Read the model definition and answer for the solid it produces. Units are mm, in the model's axes. A direction names the side the tool comes from. Round coordinates to 2 decimals unless told otherwise and drop trailing zeros. Write each loop counter-clockwise with the first axis right and the second up, starting at its lowest first coordinate (ties: lowest second). Pieces come first, ordered by that corner, then holes. Notation, with made-up numbers: (42, 56.25) - (101, 56.25) arc R21 ccw to (101, 72.25) - close; hole circle Ø6 at (-33.75, -0.75). An arc over 180 degrees is marked (long way). Use one line per item in the form item = value. Start each with the question number.
1) Consider line 1 along X through (y, z) = (44.5, -8.5); line 2 along Y through (x, z) = (41, 7.25); line 3 along X through (y, z) = (43, 2.5). Determine where each line is inside the solid, lowest interval first. Write a range as from..to.
2) For faces 5 (the face through (8, 11, -4)), 6 (the face through (20, 57, 7)), 7 (the face through (32, 11, -4)), 8 (the face through (30, 6, 4)), 9 (the face through (28.11, 47.03, -1.64)), determine the directions among +Z, -Z, +X, -X, +Y, -Y from which every point of the face is accessible in a straight line to the end or side of a thin tool.
3) The part is cut by section A-A, the plane z = 8.25. Give the vertices of the cut face in (x, y).
4) Each of these flat-tipped pins is pushed along its axis until it touches: pin 1 (10 mm diameter, centred on y = 27, z = -4.5, fed in from +X); pin 2 (12 mm diameter, centred on x = 39, y = 54, fed in from -Z); pin 3 (17.5 mm diameter, centred on x = 23.5, y = 32, fed in from +Z). Where does it stop, or does it pass through?
5) For a pull along Y with two mould halves and no side action, classify faces 1 (the face through (30.78, 35.27, -8.04)), 2 (the face through (19.9, 0, 7.2)), 3 (the face through (20, 60, 8)), 4 (the face through (20, 3, 7)) as released by +Y, released by -Y, zero draft, split by the parting line, or undercut.
6) The part is cut by section B-B, the plane x = -5. Count the separate pieces of the cut face and the enclosed holes in it, plus the area to 3 significant figures.
7) The part is cut by section C-C, the plane z = -6.5. Give the vertices of the cut face in (x, y).
from build123d import *

# Parameters (mm, degrees)
CYLINDER002003_R     = 2
CYLINDER002003_DEPTH = 30
CYLINDER002004_R     = 3
CYLINDER002004_DEPTH = 11
CYLINDER_W           = 10
CYLINDER_H           = 31
CYLINDER_ANGLE       = 180
CYLINDER_ROLL_ANGLE  = -90
CYLINDER002006_R     = 10
CYLINDER002006_DEPTH = 6
SPHERE001_ROLL_ANGLE = 1
BOX008_W             = 20
BOX008_H             = 31
BOX008_DEPTH         = 6
CYLINDER006_R        = 2
CYLINDER006_DEPTH    = 10
CYLINDER008_R        = 2
CYLINDER008_DEPTH    = 10
CYLINDER007_R        = 2
CYLINDER007_DEPTH    = 10
CYLINDER005_R        = 2
CYLINDER005_DEPTH    = 10
CYLINDER001_R        = 12
CYLINDER001_DEPTH    = 12
BOX003_W             = 24
BOX003_H             = 30
BOX003_DEPTH         = 18
BOX_W                = 60
BOX_H                = 60
BOX_DEPTH            = 3
CYLINDER002002_R     = 5
CYLINDER002002_DEPTH = 15


with BuildPart() as obj1:
    # Cylinder002003 → Cylinder002003 (new body)
    with BuildSketch(Plane(origin=(26.5, 44.5, -13), x_dir=(1, 0, 0), z_dir=(0, 0, 1))):
        Circle(CYLINDER002003_R)
    extrude(amount=CYLINDER002003_DEPTH)


with BuildPart() as schnittkegel:
    # Cone003 → Cone003 (revolve)
    with BuildSketch(Plane(origin=(20, 30.3, -5), x_dir=(1, 0, 0), z_dir=(0, -1, 0))):
        Polygon((0, 0), (10, 0), (28, 15), (0, 15), align=None)
    revolve(axis=Axis((20, 30.3, -5), (0, 0, 1)))


with BuildPart() as obj2:
    # Cylinder002004 → Cylinder002004 (new body)
    with BuildSketch(Plane(origin=(26.5, 44.5, -4), x_dir=(1, 0, 0), z_dir=(0, 0, 1))):
        Circle(CYLINDER002004_R)
    extrude(amount=CYLINDER002004_DEPTH)


with BuildPart() as zylinder:
    # Cylinder → Cylinder (revolve)
    with BuildSketch(Plane.XZ):
        with Locations((5, 15.5)):
            Rectangle(CYLINDER_W, CYLINDER_H)
    revolve(axis=Axis((0, 0, 0), (0, 0, 1)), revolution_arc=CYLINDER_ANGLE)


with BuildPart() as zylinder_1:
    # Cylinder roll: moved
    add(zylinder.part.rotate(Axis((0, 0, 0), (1, 0, 0)), CYLINDER_ROLL_ANGLE))


with BuildPart() as zylinder_2:
    # Cylinder placement: moved
    add(zylinder_1.part.moved(Location((20, -11, 1))))


with BuildPart() as zylinder014:
    # Cylinder002006 → Cylinder002006 (new body)
    with BuildSketch(Plane(origin=(20, 20, 1), x_dir=(1, 0, 0), z_dir=(0, 0, 1))):
        Circle(CYLINDER002006_R)
    extrude(amount=CYLINDER002006_DEPTH)


with BuildPart() as kugel001:
    # Sphere001 → Sphere001 (revolve)
    with BuildSketch(Plane.XZ):
        with BuildLine():
            ThreePointArc((0, -10), (10, 0), (0, 10))
            Line((0, 10), (0, -10))
        make_face()
    revolve(axis=Axis((0, 0, 0), (0, 0, 1)))


with BuildPart() as kugel001_1:
    # Sphere001 roll: moved
    add(kugel001.part.rotate(Axis((0, 0, 0), (1, 0, 0)), SPHERE001_ROLL_ANGLE))


with BuildPart() as kugel001_2:
    # Sphere001 placement: moved
    add(kugel001_1.part.moved(Location((20, 20, 1))))


with BuildPart() as obj3:
    # Box008 → Box008 (new body)
    with BuildSketch(Plane(origin=(10, -11, 1), x_dir=(1, 0, 0), z_dir=(0, 0, 1))):
        with Locations((10, 15.5)):
            Rectangle(BOX008_W, BOX008_H)
    extrude(amount=BOX008_DEPTH)

    # Fusion011: union Zylinder, Zylinder014, Kugel001
    add(zylinder_2.part)
    add(zylinder014.part)
    add(kugel001_2.part)


with BuildPart() as obj3_1:
    # Fusion011 placement: moved
    add(obj3.part.moved(Location((0, 11, 0))))


with BuildPart() as zylinder006:
    # Cylinder006 → Cylinder006 (new body)
    with BuildSketch(Plane(origin=(0, 50, 0), x_dir=(1, 0, 0), z_dir=(0, 0, 1))):
        Circle(CYLINDER006_R)
    extrude(amount=CYLINDER006_DEPTH)


with BuildPart() as zylinder008:
    # Cylinder008 → Cylinder008 (new body)
    with BuildSketch(Plane(origin=(50, 50, 0), x_dir=(1, 0, 0), z_dir=(0, 0, 1))):
        Circle(CYLINDER008_R)
    extrude(amount=CYLINDER008_DEPTH)


with BuildPart() as zylinder007:
    # Cylinder007 → Cylinder007 (new body)
    with BuildSketch(Plane(origin=(50, 0, 0), x_dir=(1, 0, 0), z_dir=(0, 0, 1))):
        Circle(CYLINDER007_R)
    extrude(amount=CYLINDER007_DEPTH)


with BuildPart() as obj4:
    # Cylinder005 → Cylinder005 (new body)
    with BuildSketch(Plane.XY):
        Circle(CYLINDER005_R)
    extrude(amount=CYLINDER005_DEPTH)

    # Fusion008: union Zylinder006, Zylinder008, Zylinder007
    add(zylinder006.part)
    add(zylinder008.part)
    add(zylinder007.part)


with BuildPart() as obj4_1:
    # Fusion008 placement: moved
    add(obj4.part.moved(Location((-5, 5.3, 2))))

    # Fusion012: union obj1, SchnittKegel, obj2, obj3
    add(obj1.part)
    add(schnittkegel.part)
    add(obj2.part)
    add(obj3_1.part)


with BuildPart() as zylinder001:
    # Cylinder001 → Cylinder001 (new body)
    with BuildSketch(Plane(origin=(20, 20, -11), x_dir=(1, 0, 0), z_dir=(0, 0, 1))):
        Circle(CYLINDER001_R)
    extrude(amount=CYLINDER001_DEPTH)


with BuildPart() as aussen:
    # Box003 → Box003 (new body)
    with BuildSketch(Plane(origin=(8, -10, -11), x_dir=(1, 0, 0), z_dir=(0, 0, 1))):
        with Locations((12, 15)):
            Rectangle(BOX003_W, BOX003_H)
    extrude(amount=BOX003_DEPTH)

    # Fusion003: union Zylinder001
    add(zylinder001.part)


with BuildPart() as aussen_1:
    # Fusion003 placement: moved
    add(aussen.part.moved(Location((0, 10, 0))))


with BuildPart() as obj5:
    # Box → Box (new body)
    with BuildSketch(Plane(origin=(-10, 0, 7), x_dir=(1, 0, 0), z_dir=(0, 0, 1))):
        with Locations((30, 30)):
            Rectangle(BOX_W, BOX_H)
    extrude(amount=BOX_DEPTH)


with BuildPart() as wall:
    # Cone001 → Cone001 (revolve)
    with BuildSketch(Plane(origin=(20, 30, -5), x_dir=(1, 0, 0), z_dir=(0, -1, 0))):
        Polygon((0, 0), (12, 0), (30, 15), (0, 15), align=None)
    revolve(axis=Axis((20, 30, -5), (0, 0, 1)))

    # Fusion: union obj5
    add(obj5.part)

    # Fusion006: union aussen
    add(aussen_1.part)


with BuildPart() as fanduct:
    # Cylinder002002 → Cylinder002002 (new body)
    with BuildSketch(Plane(origin=(26.5, 44.5, -11), x_dir=(1, 0, 0), z_dir=(0, 0, 1))):
        Circle(CYLINDER002002_R)
    extrude(amount=CYLINDER002002_DEPTH)

    # Fusion013: union Wall
    add(wall.part)

    # Cut: cut obj4
    add(obj4_1.part, mode=Mode.SUBTRACT)


solid = fanduct.part
Geometry results:
q1.line_1 = 21.5..24.5, 28.5..31.5
q1.line_2 = 0..17.3, 43.3..60
q1.line_3 = 3.51..5.87, 34.13..36.49
q2.face_5 = -Z, -X, -Y
q2.face_6 = -Z
q2.face_7 = -Z, +X, -Y
q2.face_8 = -Y
q2.face_9 = +Z
q3.outline = (-10, 0) - (50, 0) - (50, 60) - (-10, 60) - close; hole circle Ø4 at (-5, 5.3); hole circle Ø4 at (-5, 55.3); hole circle Ø51.8 at (20, 30.3); hole circle Ø4 at (45, 5.3); hole circle Ø4 at (45, 55.3)
q4.pin_1 = 38.4
q4.pin_2 = 5.51
q4.pin_3 = -2.8
q5.face_1 = undercut
q5.face_2 = released by -Y
q5.face_3 = released by +Y
q5.face_4 = zero draft
q6.separate_pieces = 3
q6.enclosed_holes = 0
q6.area = 128 mm2
q7.outline = (8, 0) - (13.39, 0) - (13.39, 31) arc R6.61 cw to (26.61, 31) - (26.61, 0) - (32, 0) - (32, 30) arc R12 ccw to (27.26, 39.56) arc R5 ccw (long way) to (22.31, 41.78) arc R12 ccw to (8, 30) - close; hole circle Ø4 at (26.5, 44.5)
